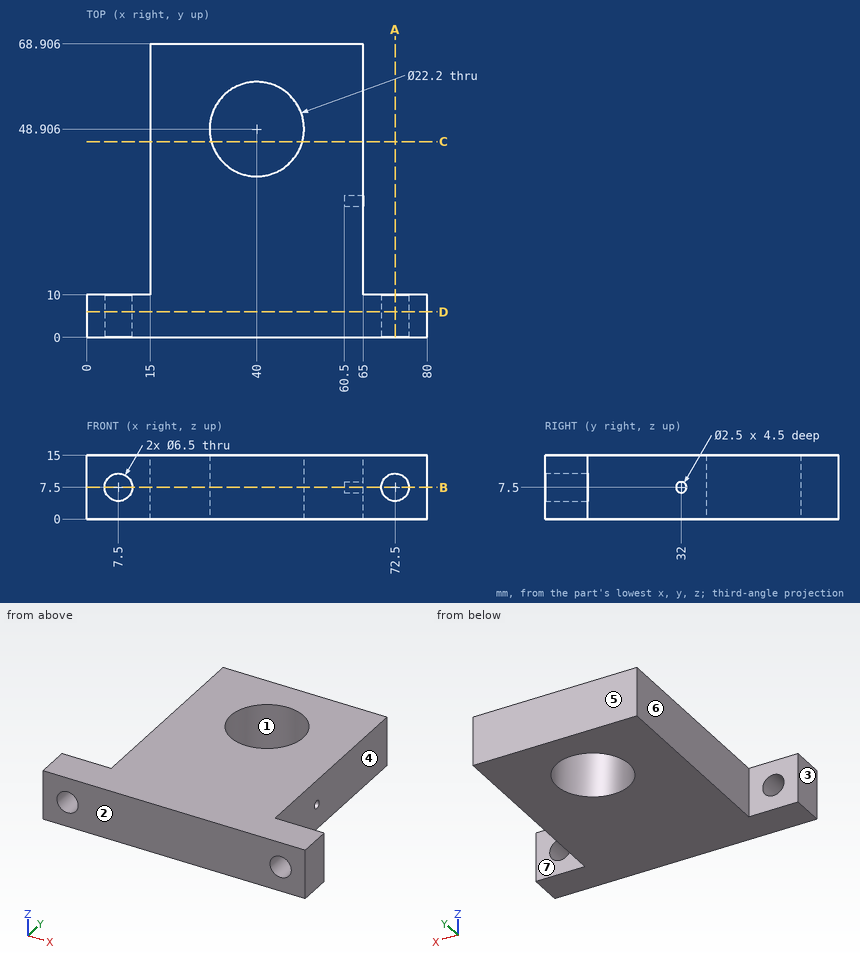
Study the drawing (mm; zero at the part's minimum x, y, z) and answer. A direction names the side the tool comes from. Give positions to 0.01 mm unless a question says otherwise; leave off trailing zeros. Order: outer loops, then holes, each group sorted by start corner. A loop starts at its lowest first (then second) coordinate and runs counter-clockwise, first axis right, second up. Notation, with made-up numbers: M -18,43.25 L 0,43.25 A28 ccw 0,75.25 Z; hole C -27.5,73.25 d2. An arc over 180 degrees is marked long. Put each result on its own line as item: value. Start each with the question number.
Item 1: The part is cut by section C-C, the plane y = 46. Determine the outline of the cut face in (x, z).
Item 2: Which of the six approach directions +Z, -Z, +X, -X, +Y, -Y give full straight-line access (tool end or side, diameter ignored) to the marked faces 5, 6 and 7?
Item 3: Flat-ended cylindrical pins translate along their axes: P1, Ø7.5, axis at x = 70.5, z = 11, coming from the +Y side; P2, Ø1, axis at y = 48.5, z = 4.5, coming from the +X side; P3, Ø0.8, axis at y = 32.5, z = 7.5, coming from the +X side; P4, Ø20, axis at x = 40, y = 48.91, coming from the -Z side. Find the tip coordinate at first contact, or state that the pin passes through.
Item 4: The part is cut by section A-A, the plane x = 72.5. Determine the outline of the cut face in (y, z).
Item 5: Find the intervals of material crossed by line 1 along Z through (x, y) = (72.5, 3.75); line 2 along Z through (x, y) = (63.15, 32); line 3 along X through (y, z) = (23.5, 7.75), in increasing order.
Item 6: The part is cut by section D-D, the plane y = 6. Determine the outline of the cut face in (x, z), and give its area (3 significant figures).
Item 7: The part is cut by section B-B, the plane z = 7.5. State how many separate pieces and enclosed holes the cut face has, and give its area (3 significant figures).
Item 8: For a pull along X with two mould halves and no side action, classify the marked faces 1, 2, 3 and 4 as +X half, -X half, draft (parallel to the pull), parting line (faces both ways), or undercut.
Answer key:
1. outline: M 15,0 L 29.29,0 L 29.29,15 L 15,15 Z; M 50.71,0 L 65,0 L 65,15 L 50.71,15 Z
2. face 5: +Z, -Z, +X, -X, +Y
2. face 6: +Z, -Z, -X, +Y
2. face 7: +Z, -Z, +X, +Y
3. P1: stops at y = 10
3. P2: stops at x = 65
3. P3: stops at x = 60.5
3. P4: passes through
4. outline: M 0,0 L 10,0 L 10,4.25 L 0,4.25 Z; M 0,10.75 L 10,10.75 L 10,15 L 0,15 Z
5. line 1: z = 0 to 4.25, 10.75 to 15
5. line 2: z = 0 to 6.25, 8.75 to 15
5. line 3: x = 15 to 65
6. outline: M 0,0 L 80,0 L 80,15 L 0,15 Z; hole C 7.5,7.5 d6.5; hole C 72.5,7.5 d6.5
6. area: 1,130 mm²
7. separate pieces: 3
7. enclosed holes: 1
7. area: 3,220 mm²
8. face 1: undercut
8. face 2: draft
8. face 3: -X half
8. face 4: +X half
